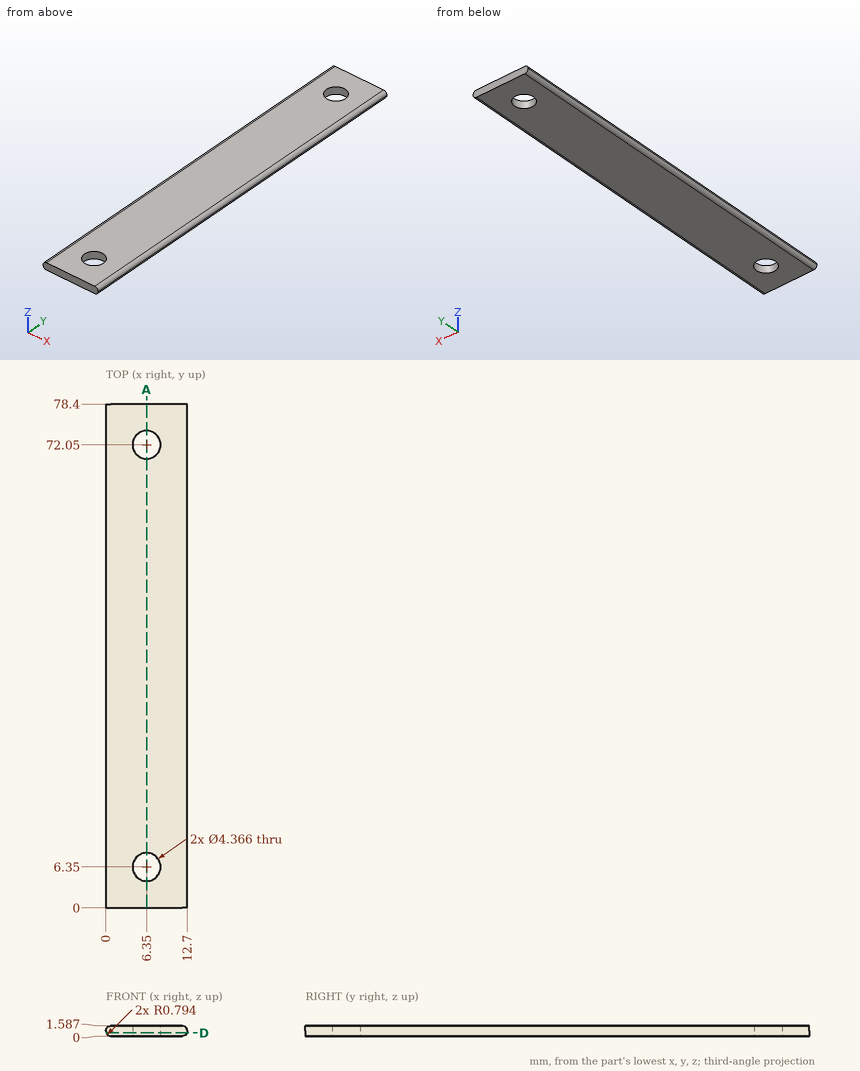
Geometry check sheet. Reference: drawing and pictorial views, mm from the part's lowest x, y, z. Round coordinates to 2 decimals unless told otherwise and drop trailing zeros. Loops run counter-clockwise (first coordinate to the right, second up) from the corner with the lowest first, then second, coordinate; pieces in that order, holes last. Notation, with made-up numbers: (48.5, 13.25) -> (89.5, 13.25) arc R23 ccw to (89.5, 23.25) -> close; hole circle Ø11 at (-12, -18.75). An arc over 180 degrees is marked (long way). Answer as a JSON object with one key per item and string values. Group by question number.
Item 1: Cross-section at D-D, the plane z = 0.5. Count the separate pieces of the cut face and the enclosed holes in it, plus the area to 3 significant figures.
Item 2: Cross-section at A-A, the plane x = 6.35. Record the cut outline in (y, z).
Item 3: Thickness scan on line 1 along Y through (x, z) = (6.35, 0.4); line 2 along Y through (x, z) = (5.5, 0.5); line 3 along Z through (x, y) = (12, 21.5) (1 decimal). Record the ranges inside material, lowest first.
Determined:
{
 "1": {"separate pieces": "1", "enclosed holes": "2", "area": "957 mm²"},
 "2": {"outline": "(0, 0) -> (4.17, 0) -> (4.17, 1.59) -> (0, 1.59) -> close; (8.53, 0) -> (69.87, 0) -> (69.87, 1.59) -> (8.53, 1.59) -> close; (74.23, 0) -> (78.4, 0) -> (78.4, 1.59) -> (74.23, 1.59) -> close"},
 "3": {"line 1": "y = 0 to 4.17, 8.53 to 69.87, 74.23 to 78.4", "line 2": "y = 0 to 4.34, 8.36 to 70.04, 74.06 to 78.4", "line 3": "z = 0 to 1.6"}
}
